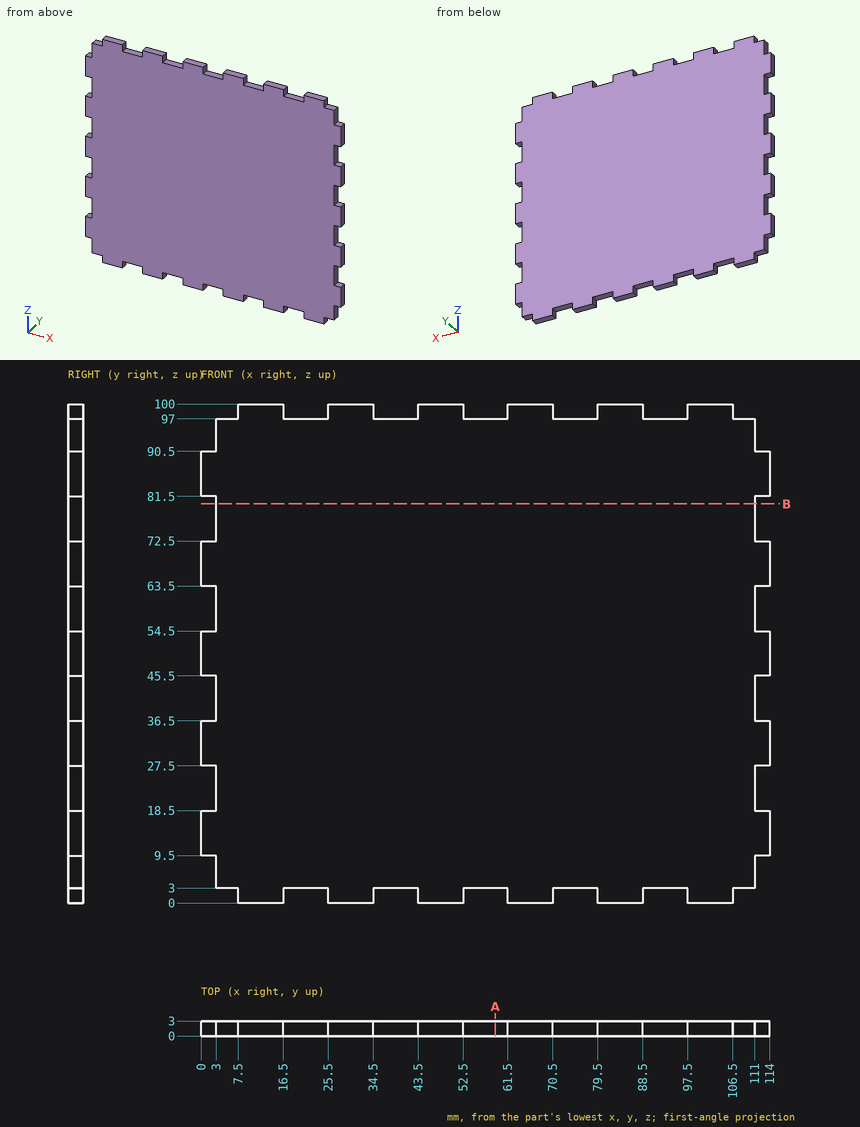
Can you work these out from the drawing? Everything is in mm from the part's minimum corner. Round coordinates to 2 decimals unless told otherwise and drop trailing zeros. Write each loop counter-clockwise with the first axis right and the second up, starting at its lowest first coordinate (ties: lowest second). Pieces come first, ordered by that corner, then holes. Notation, with made-up numbers: (-36.5, -32) - (-19.5, -32) arc R21 cw to (-19.5, -22) - close; hole circle Ø1 at (-37, 52). An arc over 180 degrees is marked (long way). Use a Markdown table: item, result.
Q1. I want a section at A-A (x = 59). List the corners of the cut face in (y, z) for me, plus the area to 3 significant figures.
Output values:
| item | result |
|---|---|
| outline | (0, 3) - (3, 3) - (3, 97) - (0, 97) - close |
| area | 282 mm2 |
Q2. For pin 1 (1.5 mm diameter, centred on y = 1, z = 41.5, fed in from -X); pin 2 (0.9 mm diameter, centred on x = 6.5, y = 1.5, fed in from +Z); pin 3 (0.9 mm diameter, centred on x = 2, y = 1.5, fed in from -Z), each with a flat end and sliding along its axis, tell me the tip position at first contact or that it passes through.
Output values:
| item | result |
|---|---|
| pin 1 | x = 3 |
| pin 2 | z = 97 |
| pin 3 | z = 9.5 |
Q3. I want a section at B-B (z = 80). List the corners of the cut face in (x, y) for me, plus the area to 3 significant figures.
Output values:
| item | result |
|---|---|
| outline | (3, 0) - (111, 0) - (111, 3) - (3, 3) - close |
| area | 324 mm2 |
Q4. Please list where these lines run through material, in increasing order: L1, parallel to Z at x = 93, y = 1.8; L2, parallel to X at y = 2.5, z = 26.5.
Output values:
| item | result |
|---|---|
| L1 | 3 to 97 |
| L2 | 3 to 111 |
